```python
from build123d import *

# Parameters (mm, degrees)
EXTRUDE_1_DEPTH     = 75
SKETCH_2_R          = 2.75
CUT_EXTRUDE_1_DEPTH = 75


with BuildPart() as part:
    # 草图1 → 凸台-拉伸1 (new body)
    with BuildSketch(Plane.XY):
        with BuildLine():
            Line((-24.396183973, 2.4), (-2.946183973, 2.4))
            ThreePointArc((-2.946183973, 2.4), (-2.687005769, -2.687005769), (2.4, -2.946183973))
            Line((2.4, -2.946183973), (2.4, -24.396183973))
            Line((2.4, -24.396183973), (3.8, -24.396183973))
            Line((3.8, -24.396183973), (3.8, 0))
            ThreePointArc((3.8, 0), (2.687005769, 2.687005769), (0, 3.8))
            Line((0, 3.8), (-24.396183973, 3.8))
            Line((-24.396183973, 3.8), (-24.396183973, 2.4))
        make_face()
    extrude(amount=EXTRUDE_1_DEPTH)

    # 草图2 → 切除-拉伸1 (cut)
    with BuildSketch(Plane(origin=(0, 3.8, 0), x_dir=(1, 0, 0), z_dir=(0, 1, 0))):
        with Locations(Location((-14.396183973, -8.5, 0), (0, 0, 180))):
            Circle(SKETCH_2_R)
        with Locations(Location((-14.396183973, -66.5, 0), (0, 0, 180))):
            Circle(SKETCH_2_R)
    cut_extrude_1 = extrude(amount=-CUT_EXTRUDE_1_DEPTH, mode=Mode.SUBTRACT)

    # 镜向1: 切除-拉伸1 across plane
    add(cut_extrude_1.mirror(Plane(origin=(0, 0, 0), x_dir=(0, 0, 1), z_dir=(-0.7071067811865488, 0.7071067811865464, 0))), mode=Mode.SUBTRACT)


solid = part.part
```
Work out the finished part from the listing and answer in its coordinate system (mm). Give positions to 0.01 mm unless a question says otherwise; leave off trailing zeros. Write each loop counter-clockwise with the first axis right and the second up, starting at its lowest first coordinate (ties: lowest second). Pieces come first, ordered by that corner, then holes. Notation, with made-up numbers: (45, -27.5) -> (74, -27.5) arc R25 ccw to (74, -12.5) -> close; hole circle Ø5 at (-2.75, -13). An arc over 180 degrees is marked (long way). Write each question's results on one line, items separated by ' | '.
1. Find section C-C on x = -4.75. Determine the outline of the cut face in (y, z), and give its area (3 significant figures).
Data:
outline: (2.4, 0) -> (3.8, 0) -> (3.8, 75) -> (2.4, 75) -> close | area: 105 mm^2
2. Find section B-B on z = 8.5. Determine the outline of the cut face in (x, y).
Data:
outline: (-24.4, 2.4) -> (-17.15, 2.4) -> (-17.15, 3.8) -> (-24.4, 3.8) -> close; (-11.65, 2.4) -> (-2.95, 2.4) arc R3.8 ccw to (2.4, -2.95) -> (2.4, -11.65) -> (3.8, -11.65) -> (3.8, 0) arc R3.8 ccw to (0, 3.8) -> (-11.65, 3.8) -> close; (2.4, -24.4) -> (3.8, -24.4) -> (3.8, -17.15) -> (2.4, -17.15) -> close
3. Determine the mould class of faces 1 (the cylindrical face through (3.11, -12.37, 10.36)), 2 (the flat face through (-2, -3, 0)), 3 (the flat face through (2.4, -14, 37)), 4 (the cylindrical face through (-12.37, 3.11, 10.36)) for opening direction Z: +Z half, -Z half, draft (parallel to the pull), parting line (faces both ways), or undercut.
Data:
face 1: undercut | face 2: -Z half | face 3: draft | face 4: undercut
4. Find section A-A on y = -14.5. Determine the outline of the cut face in (x, z).
Data:
outline: (2.4, 0) -> (3.8, 0) -> (3.8, 5.75) -> (2.4, 5.75) -> close; (2.4, 11.25) -> (3.8, 11.25) -> (3.8, 63.75) -> (2.4, 63.75) -> close; (2.4, 69.25) -> (3.8, 69.25) -> (3.8, 75) -> (2.4, 75) -> close
5. Each of these flat-tipped pins is pushed along its axis until it touches: pin 1 Ø5 at (y, z) = (-14.4, 66.5) entering from -X; pin 2 Ø7 at (x, z) = (-14.4, 66.5) entering from -Y; pin 3 Ø6.5 at (y, z) = (-14.4, 8.5) entering from -X; pin 4 Ø2 at (x, z) = (-3.5, 40) entering from -Y. Where does it stop, or does it pass through?
Data:
pin 1: through | pin 2: y = 2.4 | pin 3: x = 2.4 | pin 4: y = -2.86
6. Straight lines are drawn through the part: L1, parallel to Y at x = -22.75, z = 12.5; L2, parallel to Y at x = 3.15, z = 66.5. For each, find the intervals that lie inside material, in ascending order.
Data:
L1: 2.4 to 3.8 | L2: -24.4 to -17.15, -11.65 to 2.13
